from build123d import *

# Parameters (mm, degrees)
SKETCH1_W           = 50.8
SKETCH1_H           = 3.175
BOSS_EXTRUDE1_DEPTH = 25.4
SKETCH2_R           = 6.35
SKETCH2_R_2         = 3.175
BOSS_EXTRUDE2_DEPTH = 5.08
LPATTERN1_COUNT     = 3
LPATTERN1_PITCH     = 10.16


with BuildPart() as part:
    # Sketch1 → Boss-Extrude1 (new body)
    with BuildSketch(Plane(origin=(0, 0, 0), x_dir=(1, 0, 0), z_dir=(0, 1, 0))):
        with Locations((25.4, 1.5875)):
            Rectangle(SKETCH1_W, SKETCH1_H)
    extrude(amount=BOSS_EXTRUDE1_DEPTH)

    # Sketch2 → Boss-Extrude2 (add)
    with BuildSketch(Plane(origin=(0, 25.4, 0), x_dir=(1, 0, 0), z_dir=(0, 1, 0))):
        with Locations((50.8, 6.35)):
            Circle(SKETCH2_R)
        with Locations(Location((50.8, 6.35, 0), (0, 0, 270))):
            Circle(SKETCH2_R_2, mode=Mode.SUBTRACT)
    boss_extrude2 = extrude(amount=-BOSS_EXTRUDE2_DEPTH)

    # LPattern1: Boss-Extrude2 ×3
    with Locations(*[(0, -i * LPATTERN1_PITCH, 0) for i in range(1, LPATTERN1_COUNT)]):
        add(boss_extrude2)


solid = part.part
Can you work these out from the model? Positions are in its coordinate system, mm. A direction names the side the tool comes from. Round coordinates to 2 decimals unless told otherwise and drop trailing zeros. Write each loop counter-clockwise with the first axis right and the second up, starting at its lowest first coordinate (ties: lowest second). Pieces come first, ordered by that corner, then holes. Notation, with made-up numbers: (69, 71) -> (73, 71) arc R19 ccw to (73, 83) -> close; hole circle Ø11 at (0.25, 59). An arc over 180 degrees is marked (long way). One line per question, with ' | ' between items. Start each with the question number.
1) On a 3-axis mill with a long thin cutter (end or side, diameter ignored), from which of +Z, -Z, +X, -X, +Y, -Y can I reach the whole of each face in a straight line? I mean faces 5 (the cylindrical face through (53.95, 12.74, -6.76)), 6 (the flat face through (54, 15.24, -9)), 7 (the flat face through (50.8, 18, -2)). Say none if no direction works.
2) I need wall thicknesses on line 1 (Y direction, x = 45.5, z = -5.5); line 2 (X direction, y = 21.45, z = -6.35) (3 decimals); line 3 (Z direction, x = 25.5, y = 17.5) (3 decimals). Which ranges of each line are inside material? Lowest first, please. Write a range as [from, to].
3) Suppose I cut it at A-A on z = -6.35. Write out the boundary of the cut face in (x, y) (3 decimals), then the cut area to 3 significant figures.
4) Suppose I cut it at D-D on x = 24.5. Write out the boundary of the cut face in (y, z) (3 decimals).
5) I'm going to push flat-ended pins straight in: P1, Ø5, axis at y = 13.5, z = -8, coming from the -X side; P2, Ø2.5, axis at y = 18, z = -1, coming from the +X side. Where does each tip first touch, or does it pass through?
6) If we mould it in two halves opening along Y, with no side actions, what happens to faces 1 (the flat face through (33, 0, -3)), 2 (the flat face through (33, 25.4, -3)), 3 (the flat face through (50.8, 8, -2)), 4 (the cylindrical face through (53.95, 22.9, -6.76))? For each: released by +Y, released by -Y, zero draft, split by the parting line, or undercut.
7) Suppose I cut it at B-B on z = -11.5. Write out the boundary of the cut face in (x, y), then the cut area to 3 significant figures.
8) Suppose I cut it at C-C on y = 3.75. Write out the boundary of the cut face in (x, z) (3 decimals), then the cut area to 3 significant figures.
Return value:
1) face 5: +Y, -Y | face 6: -Z, +X | face 7: +Z, -Z, +X
2) line 1: y = [0, 5.08], [10.16, 15.24], [20.32, 25.4] | line 2: x = [44.45, 47.625], [53.975, 57.15] | line 3: z = [-3.175, 0]
3) outline: (44.45, 0) -> (47.625, 0) -> (47.625, 5.08) -> (44.45, 5.08) -> close; (44.45, 10.16) -> (47.625, 10.16) -> (47.625, 15.24) -> (44.45, 15.24) -> close; (44.45, 20.32) -> (47.625, 20.32) -> (47.625, 25.4) -> (44.45, 25.4) -> close; (53.975, 0) -> (57.15, 0) -> (57.15, 5.08) -> (53.975, 5.08) -> close; (53.975, 10.16) -> (57.15, 10.16) -> (57.15, 15.24) -> (53.975, 15.24) -> close; (53.975, 20.32) -> (57.15, 20.32) -> (57.15, 25.4) -> (53.975, 25.4) -> close | area: 96.8 mm2
4) outline: (0, -3.175) -> (25.4, -3.175) -> (25.4, 0) -> (0, 0) -> close
5) P1: stops at x = 44.45 | P2: stops at x = 50.8
6) face 1: released by -Y | face 2: released by +Y | face 3: undercut | face 4: zero draft
7) outline: (47.09, 0) -> (54.51, 0) -> (54.51, 5.08) -> (47.09, 5.08) -> close; (47.09, 10.16) -> (54.51, 10.16) -> (54.51, 15.24) -> (47.09, 15.24) -> close; (47.09, 20.32) -> (54.51, 20.32) -> (54.51, 25.4) -> (47.09, 25.4) -> close | area: 113 mm2
8) outline: (0, -3.175) -> (45.301, -3.175) arc R6.35 ccw (long way) to (50.8, 0) -> (0, 0) -> close; hole circle Ø6.35 at (50.8, -6.35) | area: 244 mm2
